Work out the finished part from the listing and answer in its coordinate system (mm). Coordinates: 2 decimals unless noted, no trailing zeros. Write each loop counter-clockwise with the first axis right and the second up, starting at its lowest first coordinate (ties: lowest second). Pieces come first, ordered by that corner, then holes. Notation, with made-up numbers: (-10, 20.25) - (23, 20.25) arc R19 cw to (23, 46.25) - close; hole circle Ø10 at (5.5, 52). An arc over 180 degrees is marked (long way). One line per item, written item: value.
```python
from build123d import *

# Parameters (mm, degrees)
SKETCH_1_R      = 19
SKETCH_1_R_2    = 12
EXTRUDE_1_DEPTH = 11
CHAMFER_1_SIZE  = 1
SKETCH_3_W      = 3.4
SKETCH_3_H      = 19


with BuildPart() as part:
    # 草图1 → 凸台-拉伸1 (new, symmetric)
    with BuildSketch(Plane.XY):
        Circle(SKETCH_1_R)
        Circle(SKETCH_1_R_2, mode=Mode.SUBTRACT)
    extrude(amount=EXTRUDE_1_DEPTH, both=True)

    # 倒角1
    chamfer_1_edges = [part.edges().sort_by_distance(p)[0] for p in [
        (-12, 0, -11),
        (-12, 0, 11),
    ]]
    chamfer(chamfer_1_edges, length=CHAMFER_1_SIZE)

    # 草图3 → M8 螺纹孔1 (revolve, cut)
    with BuildSketch(Plane(origin=(0, 0, 0), x_dir=(0, 0, -1), z_dir=(1, 0, 0))):
        with Locations((1.7, 9.5)):
            Rectangle(SKETCH_3_W, SKETCH_3_H)
    revolve(axis=Axis((0, -6.35, 0), (0, 1, 0)), mode=Mode.SUBTRACT)


solid = part.part
```
Item 1: Section C-C, the plane z = -7.25 is taken. Determine the outline of the cut face in (x, y).
Evaluation:
outline: circle Ø38 at (0, 0); hole circle Ø24 at (0, 0)
Item 2: Section A-A, the plane x = 0 is taken. Determine the outline of the cut face in (y, z).
Evaluation:
outline: (-19, -11) - (-13, -11) - (-12, -10) - (-12, 10) - (-13, 11) - (-19, 11) - close; (12, -10) - (13, -11) - (19, -11) - (19, -3.4) - (12, -3.4) - close; (12, 3.4) - (19, 3.4) - (19, 11) - (13, 11) - (12, 10) - close
Item 3: Determine the mould class of faces 1 (the face through (1.3, 15.3, -3.14)), 2 (the face through (-4.119, -18.548, 0.154)), 3 (the face through (-4.5, -12.4, -11)) for opening direction X: +X half, -X half, draft (parallel to the pull), parting line (faces both ways), or undercut.
Evaluation:
face 1: undercut
face 2: parting line
face 3: draft
Item 4: Section D-D, the plane z = 0 is taken. Determine the outline of the cut face in (x, y), then the cut area to 3 significant figures.
Evaluation:
outline: (-3.4, 11.51) - (-3.4, 18.69) arc R19 ccw (long way) to (3.4, 18.69) - (3.4, 11.51) arc R12 cw (long way) to start
area: 634 mm2
Item 5: Consider probe 1 along X at (y, z) = (0.5, 7.75); probe 2 along Z at (x, y) = (0, 13); probe 3 along Y at (x, z) = (0, 5). Determine where each line is inside the solid, lowest interval first.
Evaluation:
probe 1: x = -18.99 to -11.99, 11.99 to 18.99
probe 2: z = -11 to -3.4, 3.4 to 11
probe 3: y = -19 to -12, 12 to 19
Item 6: Given pin 1 (21.5 mm diameter, centred on x = 0, y = 0, fed in from -Z); pin 2 (1 mm diameter, centred on x = -4.5, z = 3, fed in from +Y); pin 3 (1 mm diameter, centred on y = 10.5, z = -5.5, fed in from -X); pin 4 (2 mm diameter, centred on x = 14.5, z = 4, fed in from -Y), each flat-ended and moving along its own axis, determine where each tip first touches the part or whether it passes through.
Evaluation:
pin 1: passes through
pin 2: stops at y = 18.57
pin 3: stops at x = -16.16
pin 4: stops at y = -13.37
Item 7: Section B-B, the plane y = 0 is taken. Determine the outline of the cut face in (x, z), then the cut area to 3 significant figures.
Evaluation:
outline: (-19, -11) - (-13, -11) - (-12, -10) - (-12, 10) - (-13, 11) - (-19, 11) - close; (12, -10) - (13, -11) - (19, -11) - (19, 11) - (13, 11) - (12, 10) - close
area: 306 mm2
